The figure shows three views and two pictorial views of one solid part (mm, origin at its lowest corner). Answer the questions. A direction names the side the tool comes from. Coordinates: 2 decimals unless noted, no trailing zeros. Order: outer loops, then holes, each group sorted by start corner. A loop starts at its lowest first (then second) coordinate and runs counter-clockwise, first axis right, second up. Notation, with made-up numbers: (31, 52) -> (58, 52) arc R20 cw to (58, 80) -> close; hole circle Ø8 at (-39.5, -20.75). An arc over 180 degrees is marked (long way). Return JSON: item names as keys, results as strings.
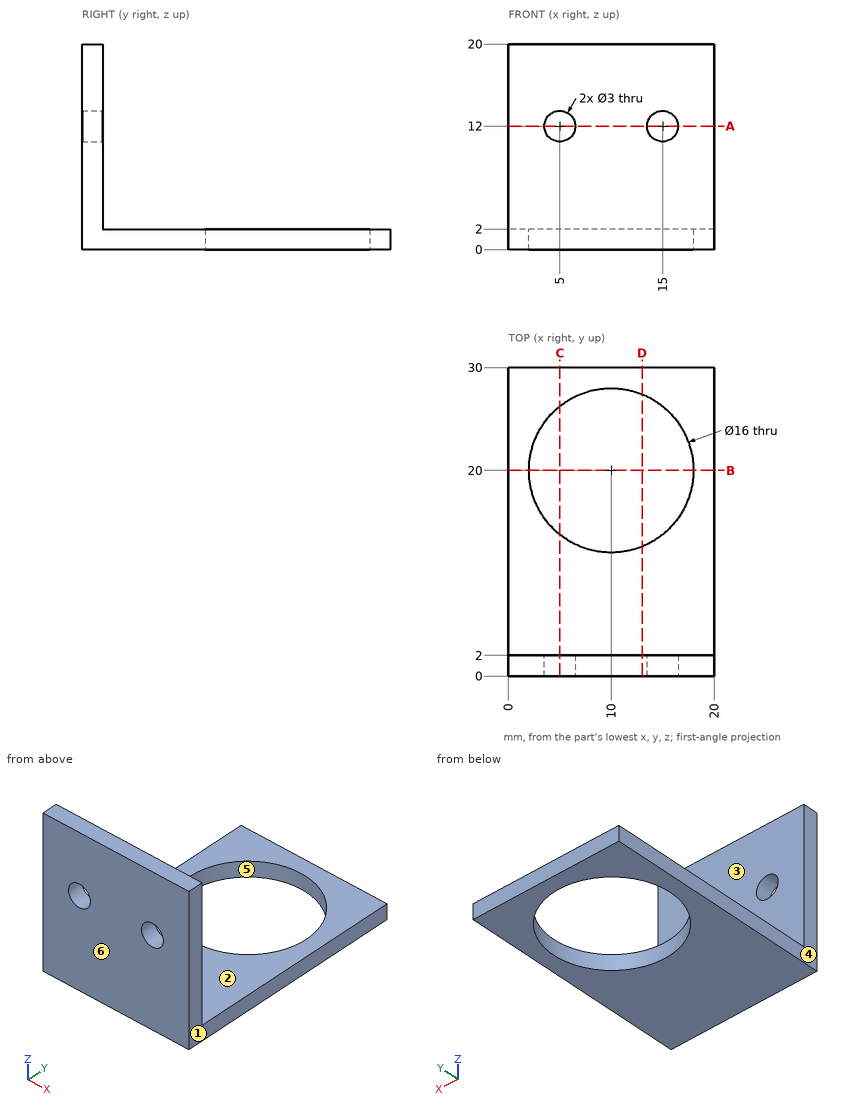
1. For the marked faces 1 and 2, determine the directions among +Z, -Z, +X, -X, +Y, -Y from which every point of the face is accessible in a straight line to the end or side of a thin tool.
Answer block:
{"face 1": "+Z, -Z, +X, +Y, -Y", "face 2": "+Z, +X, -X, +Y"}
2. Consider line 1 (X direction, y = 0.55, z = 12); line 2 (Z direction, x = 15, y = 0.5); line 3 (Z direction, x = 16, y = 10). Determine where each line is inside the solid, lowest interval first. Write a range as from..to.
Answer block:
{"line 1": "x = 0..3.5, 6.5..13.5, 16.5..20", "line 2": "z = 0..10.5, 13.5..20", "line 3": "z = 0..2"}
3. Determine the mould class of the marked faces 3, 4, 5 and 6 for opening direction Y: pulls with the +Y half, pulls with the -Y half, needs draft (parallel to the pull), parting line crosses it, or undercut.
Answer block:
{"face 3": "pulls with the +Y half", "face 4": "needs draft", "face 5": "undercut", "face 6": "pulls with the -Y half"}
4. The part is cut by section D-D on x = 13. Give the vertices of the cut face in (y, z).
Answer block:
{"outline": "(0, 0) -> (12.58, 0) -> (12.58, 2) -> (2, 2) -> (2, 20) -> (0, 20) -> close; (27.42, 0) -> (30, 0) -> (30, 2) -> (27.42, 2) -> close"}
5. Each of these flat-tipped pins is pushed along its axis until it touches: pin 1 Ø1.8 at (x, z) = (5, 12) entering from +Y; pin 2 Ø2 at (x, z) = (7, 8) entering from +Y; pin 3 Ø2 at (x, z) = (12.5, 4) entering from -Y. Where does it stop, or does it pass through?
Answer block:
{"pin 1": "passes through", "pin 2": "stops at y = 2", "pin 3": "stops at y = 0"}
6. The part is cut by section B-B on y = 20. Give the vertices of the cut face in (x, z).
Answer block:
{"outline": "(0, 0) -> (2, 0) -> (2, 2) -> (0, 2) -> close; (18, 0) -> (20, 0) -> (20, 2) -> (18, 2) -> close"}
7. The part is cut by section A-A on z = 12. Give the vertices of the cut face in (x, y).
Answer block:
{"outline": "(0, 0) -> (3.5, 0) -> (3.5, 2) -> (0, 2) -> close; (6.5, 0) -> (13.5, 0) -> (13.5, 2) -> (6.5, 2) -> close; (16.5, 0) -> (20, 0) -> (20, 2) -> (16.5, 2) -> close"}
8. The part is cut by section C-C on x = 5. Give the vertices of the cut face in (y, z) (3 decimals), and give its area (3 significant figures).
Answer block:
{"outline": "(0, 0) -> (13.755, 0) -> (13.755, 2) -> (2, 2) -> (2, 10.5) -> (0, 10.5) -> close; (0, 13.5) -> (2, 13.5) -> (2, 20) -> (0, 20) -> close; (26.245, 0) -> (30, 0) -> (30, 2) -> (26.245, 2) -> close", "area": "65.0 mm2"}
